from build123d import *

# Parameters (mm, degrees)
SKETCH1_R           = 16.078
SKETCH1_R_2         = 14.478
BOSS_EXTRUDE1_DEPTH = 3.302
SKETCH2_R           = 1.5875
CUT_EXTRUDE1_DEPTH  = 33.156
BOSS_EXTRUDE2_START = -0.635
SKETCH3_R           = 1.5875
BOSS_EXTRUDE2_DEPTH = 3.81
CIRPATTERN1_COUNT   = 2


with BuildPart() as part:
    # Sketch1 → Boss-Extrude1 (new body)
    with BuildSketch(Plane.XY):
        Circle(SKETCH1_R)
        Circle(SKETCH1_R_2, mode=Mode.SUBTRACT)
    extrude(amount=BOSS_EXTRUDE1_DEPTH)

    # Sketch2 → Cut-Extrude1 (cut, through all)
    with BuildSketch(Plane(origin=(16.078, 0, 0), x_dir=(0, 0, -1), z_dir=(1, 0, 0))):
        with Locations((-1.651, 0)):
            Circle(SKETCH2_R)
    extrude(amount=-CUT_EXTRUDE1_DEPTH, mode=Mode.SUBTRACT)

    # Sketch3 → Boss-Extrude2 (add)
    with BuildSketch(Plane(origin=(0, 16.078, 0), x_dir=(-1, 0, 0), z_dir=(0, 1, 0)).offset(BOSS_EXTRUDE2_START)):
        with Locations(Location((0, 1.651, 0), (0, 0, 90))):  # turned: the seam where the file's is
            Circle(SKETCH3_R)
    boss_extrude2 = extrude(amount=BOSS_EXTRUDE2_DEPTH)

    # CirPattern1: Boss-Extrude2 ×2 about axis
    cirpattern1_axis = Axis((0, 0, 3.302), (0, 0, -1))
    for i in range(1, CIRPATTERN1_COUNT):
        add(boss_extrude2.rotate(cirpattern1_axis, i * 360 / CIRPATTERN1_COUNT))


solid = part.part
Can you work these out from the model? Positions are in its coordinate system, mm. A direction names the side the tool comes from. Coordinates: 2 decimals unless noted, no trailing zeros. Write each loop counter-clockwise with the first axis right and the second up, starting at its lowest first coordinate (ties: lowest second). Pieces come first, ordered by that corner, then holes. Notation, with made-up numbers: (11, 18.5) -> (23, 18.5) arc R33 cw to (23, 48.5) -> close; hole circle Ø11 at (28.25, 49). An arc over 180 degrees is marked (long way). Write each question's results on one line, items separated by ' | '. Start each with the question number.
Q1. I'm going to push flat-ended pins straight in: pin 1 (1 mm diameter, centred on x = -4, z = 0.5, fed in from +Y); pin 2 (6 mm diameter, centred on x = 11.5, y = -13, fed in from -Z); pin 3 (1.5 mm diameter, centred on y = -11, z = 1.5, fed in from +X). Where does each tip first touch, or does it pass through?
Q2. If I drill on probe 1 along Y at (x, z) = (0, 2.2); probe 2 along X at (y, z) = (-12, 0.95); probe 3 along X at (y, z) = (6.5, 1.35), over which ranges is the centre line in solid material (lowest first)?
Q3. On a 3-axis mill with a long thin cutter (end or side, diameter ignored), from which of +Z, -Z, +X, -X, +Y, -Y can I reach the whole of each face in a straight line? I mean faces 1 (the face through (0.608, -17.603, 3.117)), 2 (the face through (0.477, 17.603, 3.165)), 3 (the face through (0, -19.253, 2)). Say none if no direction works.
Q4. Imagine slicing it at C-C (y = 5.5). Write out the boundary of the cut face in (x, z).
Q5. Imagine slicing it at A-A (x = 0). Write out the boundary of the cut face in (y, z), then the cut area to 3 significant figures.
Q6. Imagine slicing it at B-B (y = 0). Write out the boundary of the cut face in (x, z), then the cut area to 3 significant figures.
Q7. Imagine slicing it at D-D (z = 0.75). Write out the boundary of the cut face in (x, y), then the cut area to 3 significant figures.
Q8. We'd pull the mould along X, two halves only. Please class faces 4 (the face through (14.85, -6.16, 1.63)), 5 (the face through (-12, 8.4, 0)), 6 (the face through (13.81, 4.35, 1.63)): +X half, -X half, draft (parallel to the pull), parting line (faces both ways), or undercut.
Taken from the geometry:
1) pin 1: stops at y = 15.69 | pin 2: stops at z = 0 | pin 3: stops at x = 12.39
2) probe 1: y = -19.25 to -14.48, 14.48 to 19.25 | probe 2: x = -10.7 to -8.1, 8.1 to 10.7 | probe 3: x = -14.71 to -12.94, 12.94 to 14.71
3) face 1: -Y | face 2: +Y | face 3: +Z, -Z, +X, -X, -Y
4) outline: (-15.11, 0) -> (-13.39, 0) -> (-13.39, 3.3) -> (-15.11, 3.3) -> close; (13.39, 0) -> (15.11, 0) -> (15.11, 3.3) -> (13.39, 3.3) -> close
5) outline: (-19.25, 0.06) -> (-16.08, 0.06) -> (-16.08, 0) -> (-14.48, 0) -> (-14.48, 3.3) -> (-16.08, 3.3) -> (-16.08, 3.24) -> (-19.25, 3.24) -> close; (14.48, 0) -> (16.08, 0) -> (16.08, 0.06) -> (19.25, 0.06) -> (19.25, 3.24) -> (16.08, 3.24) -> (16.08, 3.3) -> (14.48, 3.3) -> close | area: 30.7 mm^2
6) outline: (-16.08, 0) -> (-14.48, 0) -> (-14.48, 0.06) -> (-16.08, 0.06) -> close; (-16.08, 3.24) -> (-14.48, 3.24) -> (-14.48, 3.3) -> (-16.08, 3.3) -> close; (14.48, 0) -> (16.08, 0) -> (16.08, 0.06) -> (14.48, 0.06) -> close; (14.48, 3.24) -> (16.08, 3.24) -> (16.08, 3.3) -> (14.48, 3.3) -> close | area: 0.406 mm^2
7) outline: (-16.02, -1.31) arc R16.08 ccw to (-1.31, -16.02) -> (-1.31, -19.25) -> (1.31, -19.25) -> (1.31, -16.02) arc R16.08 ccw to (16.02, -1.31) -> (14.42, -1.31) arc R14.48 cw to (-14.42, -1.31) -> close; (-16.02, 1.31) -> (-14.42, 1.31) arc R14.48 cw to (14.42, 1.31) -> (16.02, 1.31) arc R16.08 ccw to (1.31, 16.02) -> (1.31, 19.25) -> (-1.31, 19.25) -> (-1.31, 16.02) arc R16.08 ccw to start | area: 162 mm^2
8) face 4: parting line | face 5: draft | face 6: undercut
